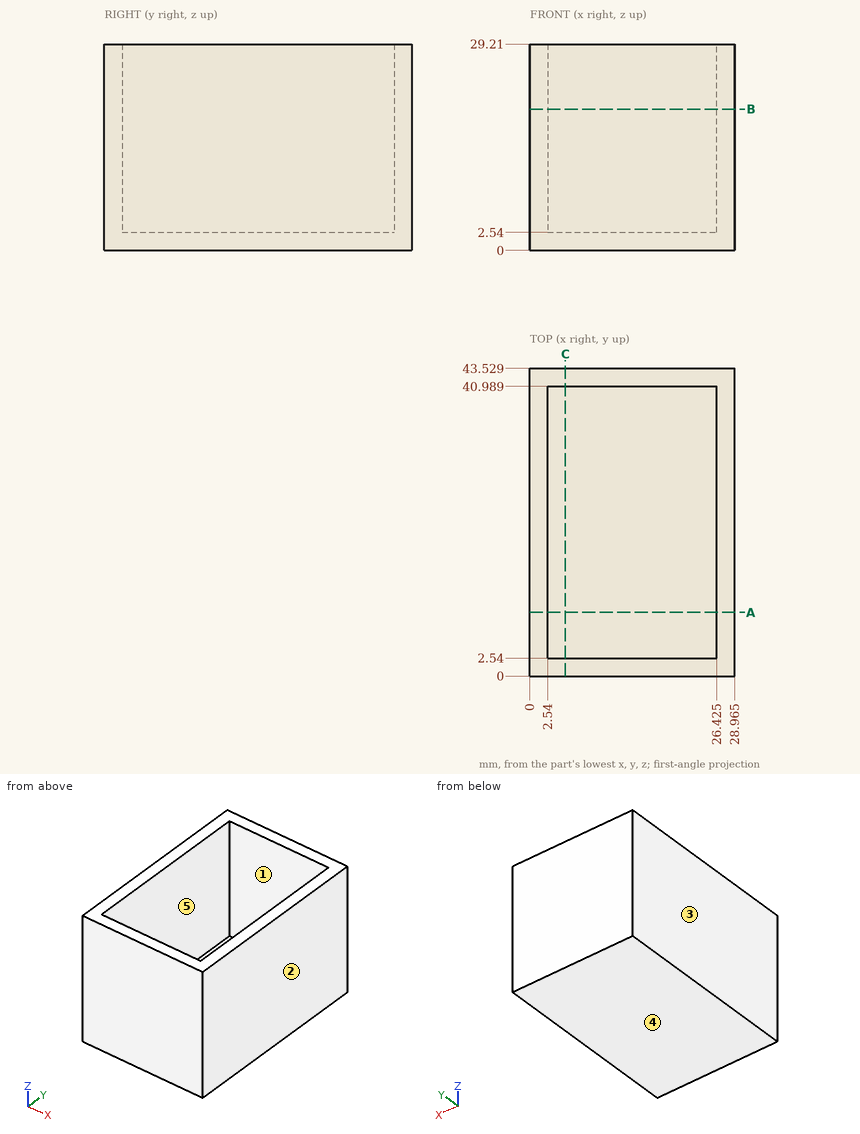
Geometry check sheet. Reference: drawing and pictorial views, mm from the part's lowest x, y, z. A direction names the side the tool comes from. Give positions to 0.01 mm unless a question says otherwise; leave off trailing zeros. Write each loop counter-clockwise with the first axis right and the second up, starting at its lowest first coordinate (ties: lowest second). Pieces come first, ordered by that corner, then holes.
Item 1: Cross-section at C-C (x = 5). Enter the section's corners in (y, z), and give its area (3 significant figures).
Item 2: Gauge pin test, flat end, axial feed: pin 1 (6 mm diameter, centred on x = 16, y = 32, fed in from +Z). Record the tip position at first contact, or that the pin passes through.
Item 3: Draft check along X on the marked faces 3, 4 and 5. Enter one of: released by +X, released by -X, zero draft, split by the parting line, or undercut.
Item 4: Access from +Z, -Z, +X, -X, +Y, -Y to the whole of each face (thin tool, end or side, straight path). Record for the marked faces 1 and 2.
Item 5: Cross-section at B-B (z = 20). Enter the section's corners in (x, y) (1 decimal).
Item 6: Cross-section at A-A (y = 9). Enter the section's corners in (x, z) (1 decimal), and give its area (3 significant figures).
Item 7: Scan lines: L1, parallel to Y at x = 22.25, z = 11; L2, parallel to X at y = 19, z = 11.25 (1 decimal); L3, parallel to Z at x = 9.25, y = 19. Record each from-to range of solid material in increasing order.
Report:
1. outline: (0, 0) - (43.53, 0) - (43.53, 29.21) - (40.99, 29.21) - (40.99, 2.54) - (2.54, 2.54) - (2.54, 29.21) - (0, 29.21) - close
1. area: 246 mm2
2. pin 1: stops at z = 2.54
3. face 3: released by -X
3. face 4: zero draft
3. face 5: undercut
4. face 1: +Z
4. face 2: +Z, -Z, +X, +Y, -Y
5. outline: (0, 0) - (29, 0) - (29, 43.5) - (0, 43.5) - close; hole (2.5, 2.5) - (26.4, 2.5) - (26.4, 41) - (2.5, 41) - close
6. outline: (0, 0) - (29, 0) - (29, 29.2) - (26.4, 29.2) - (26.4, 2.5) - (2.5, 2.5) - (2.5, 29.2) - (0, 29.2) - close
6. area: 209 mm2
7. L1: y = 0 to 2.54, 40.99 to 43.53
7. L2: x = 0 to 2.5, 26.4 to 29
7. L3: z = 0 to 2.54
